Can you work these out from the drawing? Everything is in mm from the part's minimum corner. Coordinates: 2 decimals unless noted, no trailing zeros. Loops run counter-clockwise (first coordinate to the right, second up) from the corner with the lowest first, then second, coordinate; pieces in that order, holes last.
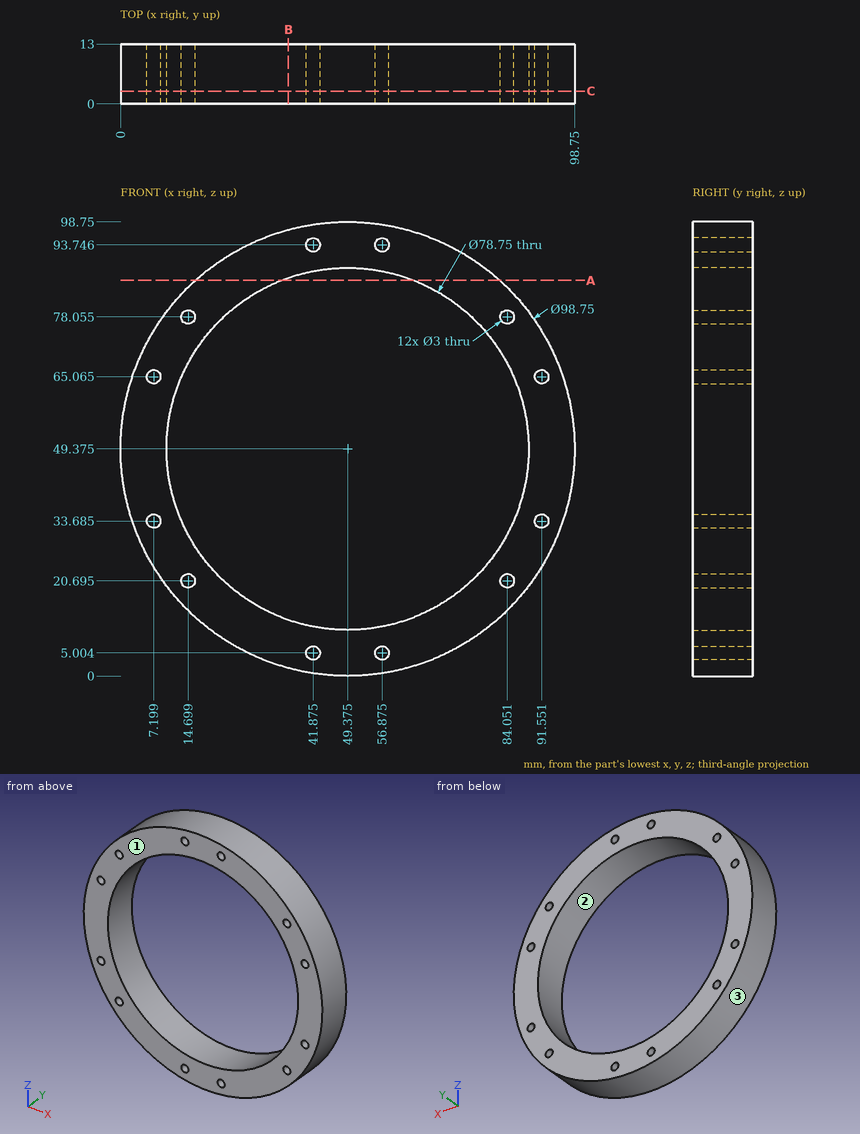
1) Imagine slicing it at A-A on z = 86. List the corners of the cut face in (x, y) for me.
2) Imagine slicing it at C-C on y = 2.75. State how many separate pieces and enclosed holes the cut face has, plus the area to 3 significant figures.
3) Will these pins go through, and if not, where does the flat tip stop? pin 1 (6 mm diameter, centred on y = 10, z = 70, fed in from -X); pin 2 (2.5 mm diameter, centred on x = 91.55, z = 33.68, fed in from -Y); pin 3 (1 mm diameter, centred on x = 35.5, y = 8, fed in from +Z); pin 4 (2 mm diameter, centred on y = 11, z = 81, fed in from +X) (1 decimal).
4) If I drill on L1, parallel to X at y = 6.75, z = 64 (1 decimal); L2, parallel to X at y = 7.25, z = 21 (1 decimal); L3, parallel to Z at x = 91.5, y = 1.5 (1 decimal), over which ranges is the centre line in solid material (lowest first)?
5) Imagine slicing it at B-B on x = 36.5. List the corners of the cut face in (y, z) for me (1 decimal).
6) We'd pull the mould along Z, two halves only. Please class the marked faces 1, 2 and 3: released by +Z, released by -Z, zero draft, split by the parting line, or undercut.
Solved:
1. outline: (16.26, 0) - (34.92, 0) - (34.92, 13) - (16.26, 13) - close; (63.83, 0) - (82.49, 0) - (82.49, 13) - (63.83, 13) - close
2. separate pieces: 1
2. enclosed holes: 13
2. area: 2,700 mm2
3. pin 1: stops at x = 3.25
3. pin 2: passes through
3. pin 3: stops at z = 96.9
3. pin 4: stops at x = 88.1
4. L1: x = 2.2 to 6.1, 8.3 to 12.8, 85.9 to 90.5, 92.6 to 96.5
4. L2: x = 9 to 13.2, 16.2 to 22.1, 76.7 to 82.6, 85.5 to 89.8
4. L3: z = 23.6 to 32.2, 35.2 to 63.6, 66.6 to 75.1
5. outline: (0, 1.7) - (13, 1.7) - (13, 12.2) - (0, 12.2) - close; (0, 86.6) - (13, 86.6) - (13, 97) - (0, 97) - close
6. face 1: zero draft
6. face 2: undercut
6. face 3: split by the parting line
